from build123d import *

# Parameters (mm, degrees)
BOSS_EXTRUDE1_DEPTH = 30
SKETCH3_R           = 7.75
CUT_EXTRUDE1_DEPTH  = 30
FILLET1_R           = 5
SKETCH4_W           = 36
SKETCH4_H           = 30
BOSS_EXTRUDE2_DEPTH = 4
SKETCH9_W           = 149
SKETCH9_H           = 30
BOSS_EXTRUDE5_DEPTH = 0.5


with BuildPart() as part:
    # Sketch2 → Boss-Extrude1 (new body)
    with BuildSketch(Plane(origin=(0, 0, 0), x_dir=(1, 0, 0), z_dir=(0, 1, 0))):
        Polygon((-14.863905325, 0), (-6.863905325, 0), (-6.863905325, 20), (13.136094675, 20), (13.136094675, 0), (21.136094675, 0), (21.136094675, -3), (-14.863905325, -3), align=None)
    extrude(amount=BOSS_EXTRUDE1_DEPTH)

    # Sketch3 → Cut-Extrude1 (cut)
    with BuildSketch(Plane.XZ):
        with Locations(Location((3.136094675, -8.5, 0), (0, 0, 270))):
            Circle(SKETCH3_R)
    extrude(amount=-CUT_EXTRUDE1_DEPTH, mode=Mode.SUBTRACT)

    # Fillet1
    fillet1_edges = [part.edges().sort_by_distance(p)[0] for p in [
        (-6.863905325, 15, -20),
        (13.136094675, 15, -20),
    ]]
    fillet(fillet1_edges, radius=FILLET1_R)

    # Sketch4 → Boss-Extrude2 (add)
    with BuildSketch(Plane.XY.offset(3)):
        with Locations((3.136094675, 15)):
            Rectangle(SKETCH4_W, SKETCH4_H)
    extrude(amount=BOSS_EXTRUDE2_DEPTH)


with BuildPart() as body_2:
    # Body-Move/Copy2: copy of part
    add(part.part.moved(Location((113, 0, 0))))


with BuildPart() as part_1:
    add(part.part)

    add(body_2.part)  # Boss-Extrude5 merges body 2
    # Sketch9 → Boss-Extrude5 (add)
    with BuildSketch(Plane.XY.offset(7)):
        with Locations((59.636094675, 15)):
            Rectangle(SKETCH9_W, SKETCH9_H)
    extrude(amount=BOSS_EXTRUDE5_DEPTH)


solid = part_1.part
Input: part model. Units: mm. Frame: model coordinates. A direction names the side the tool comes from. Coordinates: 2 decimals unless noted, no trailing zeros. Loops run counter-clockwise (first coordinate to the right, second up) from the corner with the lowest first, then second, coordinate; pieces in that order, holes last.
(1) Section D-D on x = 101. Return the cut outline in (y, z).
(2) Material intervals for probe 1 along X at (y, z) = (10.75, -8.5); probe 2 along Z at (x, y) = (3.5, 22.75); probe 3 along X at (y, z) = (21.5, -6), sorted ascending.
(3) Set-up query: faces 5 (the face through (13.136, 15, -8)), 6 (the face through (130, 15, 0)), 7 (the face through (-6.864, 15, -7)). Return all of +Z, -Z, +X, -X, +Y, -Y with unobstructed straight access to the full face (end or side cutting, diameter ignored); none if empty.
(4) First-contact query: pin 1 Ø6 at (y, z) = (17, -16) entering from -X; pin 2 Ø2 at (x, y) = (58, 9.5) entering from -Z; pin 3 Ø10 at (x, y) = (13.5, 5) entering from -Z. Flat tips, straight axial feed; report the tip coordinate or a pass-through.
(5) Section B-B on y = 17.25. Return the cut outline in (x, z).
(6) Section A-A on z = -8.5. Return the cut outline in (x, y).
(7) Section C-C on z = -18. Return the cut outline in (x, y).
(8) Pull-direction query (X, two-part tool) for faces 1 (the face through (103, 0, 1)), 2 (the face through (126.136, 15, -8)), 3 (the face through (-14.864, 15, 4)), 4 (the face through (107.562, 15.21, -18.496)); classes: released by +X, released by -X, zero draft, split by the parting line, or undercut.
Data:
1. outline: (0, 0) - (30, 0) - (30, 7.5) - (0, 7.5) - close
2. probe 1: x = -6.86 to -4.61, 10.89 to 13.14, 106.14 to 108.39, 123.89 to 126.14
2. probe 2: z = -20 to -16.24, -0.76 to 7.5
2. probe 3: x = -6.86 to -4.2, 10.47 to 13.14, 106.14 to 108.8, 123.47 to 126.14
3. face 5: -Z, +Y, -Y
3. face 6: -Z, +X, +Y, -Y
3. face 7: -Z, -X, +Y, -Y
4. pin 1: stops at x = -6.86
4. pin 2: stops at z = 7
4. pin 3: stops at z = -19.99
5. outline: (-14.86, 0) - (-6.86, 0) - (-6.86, -15) arc R5 ccw to (-1.86, -20) - (8.14, -20) arc R5 ccw to (13.14, -15) - (13.14, 0) - (21.14, 0) - (21.14, 7) - (98.14, 7) - (98.14, 0) - (106.14, 0) - (106.14, -15) arc R5 ccw to (111.14, -20) - (121.14, -20) arc R5 ccw to (126.14, -15) - (126.14, 0) - (134.14, 0) - (134.14, 7.5) - (-14.86, 7.5) - close; hole circle Ø15.5 at (3.14, -8.5); hole circle Ø15.5 at (116.14, -8.5)
6. outline: (-6.86, 0) - (-4.61, 0) - (-4.61, 30) - (-6.86, 30) - close; (10.89, 0) - (13.14, 0) - (13.14, 30) - (10.89, 30) - close; (106.14, 0) - (108.39, 0) - (108.39, 30) - (106.14, 30) - close; (123.89, 0) - (126.14, 0) - (126.14, 30) - (123.89, 30) - close
7. outline: (-5.86, 0) - (12.14, 0) - (12.14, 30) - (-5.86, 30) - close; (107.14, 0) - (125.14, 0) - (125.14, 30) - (107.14, 30) - close
8. face 1: zero draft
8. face 2: released by +X
8. face 3: released by -X
8. face 4: undercut
